Can you work these out from the model? Positions are in its coordinate system, mm. Face numbers are marked on the shaded views. A direction names the side the tool comes from. Coordinates: 2 decimals unless noted, no trailing zeros. Order: outer loops, then holes, each group sorted by start corner. A loop starts at its lowest first (then second) coordinate and runs counter-clockwise, first axis right, second up. Notation, with made-up numbers: (85, 13.5) -> (100, 13.5) arc R24 ccw to (100, 45.5) -> close; hole circle Ø11 at (83, 20.25). An arc over 180 degrees is marked (long way). Write item = value, one per line. Start each with the question number.
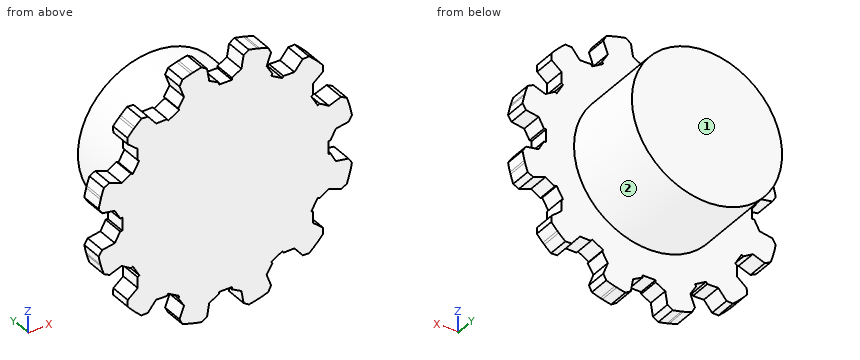
from build123d import *

# Parameters (mm, degrees)
BOSS_EXTRUDE1_DEPTH = 5
SKETCH2_R           = 17.5
BOSS_EXTRUDE3_DEPTH = 20


with BuildPart() as part:
    # Sketch1 → Boss-Extrude1 (new body)
    with BuildSketch(Plane(origin=(0, 0, 0), x_dir=(1, 0, 0), z_dir=(0, 1, 0))):
        with BuildLine():
            Line((-1.5, 24.494818027), (-3.75, 25.728146066))
            Line((-3.75, 25.728146066), (-4.25, 28.686887248))
            Line((-4.25, 28.686887248), (-5.5, 29.491524206))
            ThreePointArc((-5.5, 29.491524206), (-6.518225952, 29.283318296), (-7.528629065, 29.039968051))
            ThreePointArc((-7.528629065, 29.039968051), (-7.764571353, 28.977774789), (-8, 28.91366459))
            ThreePointArc((-8, 28.91366459), (-8.996709886, 28.619210528), (-9.982622382, 28.290409159))
            Line((-9.982622382, 28.290409159), (-10.662835658, 26.968573113))
            Line((-10.662835658, 26.968573113), (-9.616477769, 24.156228086))
            Line((-9.616477769, 24.156228086), (-10.948370908, 21.963134673))
            Line((-10.948370908, 21.963134673), (-10.700961894, 21.534609691))
            Line((-10.700961894, 21.534609691), (-13.299038106, 20.034609691))
            Line((-13.299038106, 20.034609691), (-13.546447119, 20.463134673))
            Line((-13.546447119, 20.463134673), (-16.111668297, 20.406228086))
            Line((-16.111668297, 20.406228086), (-18.02405159, 22.718573113))
            Line((-18.02405159, 22.718573113), (-19.508901824, 22.790409159))
            ThreePointArc((-19.508901824, 22.790409159), (-20.28660841, 22.100984575), (-21.039968051, 21.385035525))
            ThreePointArc((-21.039968051, 21.385035525), (-21.213203436, 21.213203436), (-21.385035525, 21.039968051))
            ThreePointArc((-21.385035525, 21.039968051), (-22.100984575, 20.28660841), (-22.790409159, 19.508901824))
            Line((-22.790409159, 19.508901824), (-22.718573113, 18.02405159))
            Line((-22.718573113, 18.02405159), (-20.406228086, 16.111668297))
            Line((-20.406228086, 16.111668297), (-20.463134673, 13.546447119))
            Line((-20.463134673, 13.546447119), (-20.034609691, 13.299038106))
            Line((-20.034609691, 13.299038106), (-21.534609691, 10.700961894))
            Line((-21.534609691, 10.700961894), (-21.963134673, 10.948370908))
            Line((-21.963134673, 10.948370908), (-24.156228086, 9.616477769))
            Line((-24.156228086, 9.616477769), (-26.968573113, 10.662835658))
            Line((-26.968573113, 10.662835658), (-28.290409159, 9.982622382))
            ThreePointArc((-28.290409159, 9.982622382), (-28.619210528, 8.996709886), (-28.91366459, 8))
            ThreePointArc((-28.91366459, 8), (-28.977774789, 7.764571353), (-29.039968051, 7.528629065))
            ThreePointArc((-29.039968051, 7.528629065), (-29.283318296, 6.518225952), (-29.491524206, 5.5))
            Line((-29.491524206, 5.5), (-28.686887248, 4.25))
            Line((-28.686887248, 4.25), (-25.728146066, 3.75))
            Line((-25.728146066, 3.75), (-24.494818027, 1.5))
            Line((-24.494818027, 1.5), (-24, 1.5))
            Line((-24, 1.5), (-24, -1.5))
            Line((-24, -1.5), (-24.494818027, -1.5))
            Line((-24.494818027, -1.5), (-25.728146066, -3.75))
            Line((-25.728146066, -3.75), (-28.686887248, -4.25))
            Line((-28.686887248, -4.25), (-29.491524206, -5.5))
            ThreePointArc((-29.491524206, -5.5), (-29.283318296, -6.518225952), (-29.039968051, -7.528629065))
            ThreePointArc((-29.039968051, -7.528629065), (-28.977774789, -7.764571353), (-28.91366459, -8))
            ThreePointArc((-28.91366459, -8), (-28.619210528, -8.996709886), (-28.290409159, -9.982622382))
            Line((-28.290409159, -9.982622382), (-26.968573113, -10.662835658))
            Line((-26.968573113, -10.662835658), (-24.156228086, -9.616477769))
            Line((-24.156228086, -9.616477769), (-21.963134673, -10.948370908))
            Line((-21.963134673, -10.948370908), (-21.534609691, -10.700961894))
            Line((-21.534609691, -10.700961894), (-20.034609691, -13.299038106))
            Line((-20.034609691, -13.299038106), (-20.463134673, -13.546447119))
            Line((-20.463134673, -13.546447119), (-20.406228086, -16.111668297))
            Line((-20.406228086, -16.111668297), (-22.718573113, -18.02405159))
            Line((-22.718573113, -18.02405159), (-22.790409159, -19.508901824))
            ThreePointArc((-22.790409159, -19.508901824), (-22.100984575, -20.28660841), (-21.385035525, -21.039968051))
            ThreePointArc((-21.385035525, -21.039968051), (-21.213203436, -21.213203436), (-21.039968051, -21.385035525))
            ThreePointArc((-21.039968051, -21.385035525), (-20.28660841, -22.100984575), (-19.508901824, -22.790409159))
            Line((-19.508901824, -22.790409159), (-18.02405159, -22.718573113))
            Line((-18.02405159, -22.718573113), (-16.111668297, -20.406228086))
            Line((-16.111668297, -20.406228086), (-13.546447119, -20.463134673))
            Line((-13.546447119, -20.463134673), (-13.299038106, -20.034609691))
            Line((-13.299038106, -20.034609691), (-10.700961894, -21.534609691))
            Line((-10.700961894, -21.534609691), (-10.948370908, -21.963134673))
            Line((-10.948370908, -21.963134673), (-9.616477769, -24.156228086))
            Line((-9.616477769, -24.156228086), (-10.662835658, -26.968573113))
            Line((-10.662835658, -26.968573113), (-9.982622382, -28.290409159))
            ThreePointArc((-9.982622382, -28.290409159), (-8.996709886, -28.619210528), (-8, -28.91366459))
            ThreePointArc((-8, -28.91366459), (-7.764571353, -28.977774789), (-7.528629065, -29.039968051))
            ThreePointArc((-7.528629065, -29.039968051), (-6.518225952, -29.283318296), (-5.5, -29.491524206))
            Line((-5.5, -29.491524206), (-4.25, -28.686887248))
            Line((-4.25, -28.686887248), (-3.75, -25.728146066))
            Line((-3.75, -25.728146066), (-1.5, -24.494818027))
            Line((-1.5, -24.494818027), (-1.5, -24))
            Line((-1.5, -24), (1.5, -24))
            Line((1.5, -24), (1.5, -24.494818027))
            Line((1.5, -24.494818027), (3.75, -25.728146066))
            Line((3.75, -25.728146066), (4.25, -28.686887248))
            Line((4.25, -28.686887248), (5.5, -29.491524206))
            ThreePointArc((5.5, -29.491524206), (6.518225952, -29.283318296), (7.528629065, -29.039968051))
            ThreePointArc((7.528629065, -29.039968051), (7.764571353, -28.977774789), (8, -28.91366459))
            ThreePointArc((8, -28.91366459), (8.996709886, -28.619210528), (9.982622382, -28.290409159))
            Line((9.982622382, -28.290409159), (10.662835658, -26.968573113))
            Line((10.662835658, -26.968573113), (9.616477769, -24.156228086))
            Line((9.616477769, -24.156228086), (10.948370908, -21.963134673))
            Line((10.948370908, -21.963134673), (10.700961894, -21.534609691))
            Line((10.700961894, -21.534609691), (13.299038106, -20.034609691))
            Line((13.299038106, -20.034609691), (13.546447119, -20.463134673))
            Line((13.546447119, -20.463134673), (16.111668297, -20.406228086))
            Line((16.111668297, -20.406228086), (18.02405159, -22.718573113))
            Line((18.02405159, -22.718573113), (19.508901824, -22.790409159))
            ThreePointArc((19.508901824, -22.790409159), (20.28660841, -22.100984575), (21.039968051, -21.385035525))
            ThreePointArc((21.039968051, -21.385035525), (21.213203436, -21.213203436), (21.385035525, -21.039968051))
            ThreePointArc((21.385035525, -21.039968051), (22.100984575, -20.28660841), (22.790409159, -19.508901824))
            Line((22.790409159, -19.508901824), (22.718573113, -18.02405159))
            Line((22.718573113, -18.02405159), (20.406228086, -16.111668297))
            Line((20.406228086, -16.111668297), (20.463134673, -13.546447119))
            Line((20.463134673, -13.546447119), (20.034609691, -13.299038106))
            Line((20.034609691, -13.299038106), (21.534609691, -10.700961894))
            Line((21.534609691, -10.700961894), (21.963134673, -10.948370908))
            Line((21.963134673, -10.948370908), (24.156228086, -9.616477769))
            Line((24.156228086, -9.616477769), (26.968573113, -10.662835658))
            Line((26.968573113, -10.662835658), (28.290409159, -9.982622382))
            ThreePointArc((28.290409159, -9.982622382), (28.619210528, -8.996709886), (28.91366459, -8))
            ThreePointArc((28.91366459, -8), (28.977774789, -7.764571353), (29.039968051, -7.528629065))
            ThreePointArc((29.039968051, -7.528629065), (29.283318296, -6.518225952), (29.491524206, -5.5))
            Line((29.491524206, -5.5), (28.686887248, -4.25))
            Line((28.686887248, -4.25), (25.728146066, -3.75))
            Line((25.728146066, -3.75), (24.494818027, -1.5))
            Line((24.494818027, -1.5), (24, -1.5))
            Line((24, -1.5), (24, 1.5))
            Line((24, 1.5), (24.494818027, 1.5))
            Line((24.494818027, 1.5), (25.728146066, 3.75))
            Line((25.728146066, 3.75), (28.686887248, 4.25))
            Line((28.686887248, 4.25), (29.491524206, 5.5))
            ThreePointArc((29.491524206, 5.5), (29.283318296, 6.518225952), (29.039968051, 7.528629065))
            ThreePointArc((29.039968051, 7.528629065), (28.977774789, 7.764571353), (28.91366459, 8))
            ThreePointArc((28.91366459, 8), (28.619210528, 8.996709886), (28.290409159, 9.982622382))
            Line((28.290409159, 9.982622382), (26.968573113, 10.662835658))
            Line((26.968573113, 10.662835658), (24.156228086, 9.616477769))
            Line((24.156228086, 9.616477769), (21.963134673, 10.948370908))
            Line((21.963134673, 10.948370908), (21.534609691, 10.700961894))
            Line((21.534609691, 10.700961894), (20.034609691, 13.299038106))
            Line((20.034609691, 13.299038106), (20.463134673, 13.546447119))
            Line((20.463134673, 13.546447119), (20.406228086, 16.111668297))
            Line((20.406228086, 16.111668297), (22.718573113, 18.02405159))
            Line((22.718573113, 18.02405159), (22.790409159, 19.508901824))
            ThreePointArc((22.790409159, 19.508901824), (22.100984575, 20.28660841), (21.385035525, 21.039968051))
            ThreePointArc((21.385035525, 21.039968051), (21.213203436, 21.213203436), (21.039968051, 21.385035525))
            ThreePointArc((21.039968051, 21.385035525), (20.28660841, 22.100984575), (19.508901824, 22.790409159))
            Line((19.508901824, 22.790409159), (18.02405159, 22.718573113))
            Line((18.02405159, 22.718573113), (16.111668297, 20.406228086))
            Line((16.111668297, 20.406228086), (13.546447119, 20.463134673))
            Line((13.546447119, 20.463134673), (13.299038106, 20.034609691))
            Line((13.299038106, 20.034609691), (10.700961894, 21.534609691))
            Line((10.700961894, 21.534609691), (10.948370908, 21.963134673))
            Line((10.948370908, 21.963134673), (9.616477769, 24.156228086))
            Line((9.616477769, 24.156228086), (10.662835658, 26.968573113))
            Line((10.662835658, 26.968573113), (9.982622382, 28.290409159))
            ThreePointArc((9.982622382, 28.290409159), (8.996709886, 28.619210528), (8, 28.91366459))
            ThreePointArc((8, 28.91366459), (7.764571353, 28.977774789), (7.528629065, 29.039968051))
            ThreePointArc((7.528629065, 29.039968051), (6.518225952, 29.283318296), (5.5, 29.491524206))
            Line((5.5, 29.491524206), (4.25, 28.686887248))
            Line((4.25, 28.686887248), (3.75, 25.728146066))
            Line((3.75, 25.728146066), (1.5, 24.494818027))
            Line((1.5, 24.494818027), (1.5, 24))
            Line((1.5, 24), (-1.5, 24))
            Line((-1.5, 24), (-1.5, 24.494818027))
        make_face()
    extrude(amount=BOSS_EXTRUDE1_DEPTH)

    # Sketch2 → Boss-Extrude3 (add)
    with BuildSketch(Plane(origin=(0, 5, 0), x_dir=(1, 0, 0), z_dir=(0, 1, 0))):
        Circle(SKETCH2_R)
    extrude(amount=BOSS_EXTRUDE3_DEPTH)


solid = part.part
(1) For the marked faces 1 and 2, which set-ups out of +Z, -Z, +X, -X, +Y, -Y let a thin tool reach every point of the face, with its end or its side?
(2) Imagine slicing it at A-A (x = 0). Write out the boundary of the cut face in (y, z).
(3) Imagine slicing it at C-C (y = 22). Write out the boundary of the cut face in (x, z), plus the area to 3 significant figures.
(4) If I drill on L1, parallel to Y at x = -19, z = -12.5; L2, parallel to X at y = 2.5, z = 0.5, over which ranges is the centre line in solid material (lowest first)? Write a range as from..to.
(5) Imagine slicing it at B-B (z = 0). Write out the boundary of the cut face in (x, y).
(6) For P1, Ø1, axis at x = -19, z = 2.5, coming from the -Y side; P2, Ø3, axis at x = -16, y = 3, coming from the +Z side; P3, Ø3, axis at x = 9, y = 9.5, coming from the +Z side; P4, Ø0.5, axis at y = 1.5, z = 24.5, coming from the -X side, each with a flat end and sliding along its axis, tell me the tip position at first contact or that it passes through.
Result set:
q1.face_1 = +Z, -Z, +X, -X, +Y
q1.face_2 = +Y
q2.outline = (0, -24) -> (5, -24) -> (5, -17.5) -> (25, -17.5) -> (25, 17.5) -> (5, 17.5) -> (5, 24) -> (0, 24) -> close
q3.outline = circle Ø35 at (0, 0)
q3.area = 962 mm2
q4.L1 = 0..5
q4.L2 = -24..24
q5.outline = (-24, 0) -> (24, 0) -> (24, 5) -> (17.5, 5) -> (17.5, 25) -> (-17.5, 25) -> (-17.5, 5) -> (-24, 5) -> close
q6.P1 = 0
q6.P2 = 22.08
q6.P3 = 15.81
q6.P4 = -9.84
